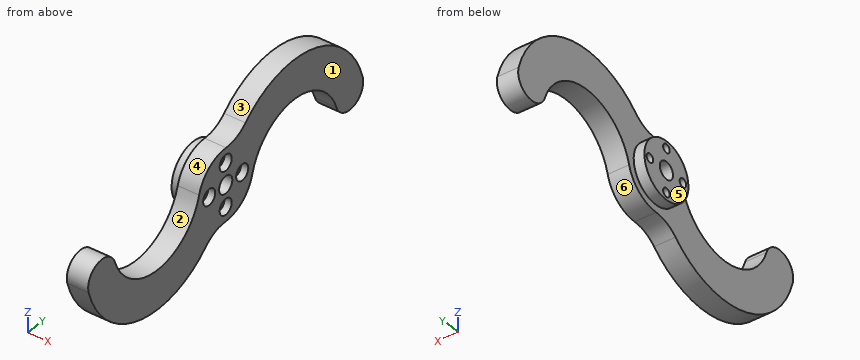
from build123d import *

# Parameters (mm, degrees)
SKETCH1_R                      = 2.4
BOSS_EXTRUDE1_DEPTH            = 6
SKETCH2_R                      = 8
SKETCH2_R_2                    = 2.4
BOSS_EXTRUDE2_DEPTH            = 3
CBORE_FOR_M2_SHCS1_D           = 2.4
CBORE_FOR_M2_SHCS1_CBORE_D     = 4.4
CBORE_FOR_M2_SHCS1_CBORE_DEPTH = 2
FILLET1_R                      = 10


with BuildPart() as part:
    # Sketch1 → Boss-Extrude1 (new body)
    with BuildSketch(Plane(origin=(0, 0, 0), x_dir=(0, 0, -1), z_dir=(1, 0, 0))):
        with BuildLine():
            ThreePointArc((9.139568575, -4.058113633), (9.024618995, 4.307696832), (2.592436286, 9.658119595))
            ThreePointArc((2.592436286, 9.658119595), (-9.251342607, 24.595099021), (1.604842351, 40.264550225))
            ThreePointArc((1.604842351, 40.264550225), (4.773868283, 46.4866715), (-1.367582481, 49.809336247))
            ThreePointArc((-1.367582481, 49.809336247), (-19.682903104, 29.384906165), (-9.139568476, 4.058113857))
            ThreePointArc((-9.139568476, 4.058113857), (-9.024618995, -4.307696832), (-2.592436049, -9.658119658))
            ThreePointArc((-2.592436049, -9.658119658), (9.25134321, -24.595098795), (-1.604841364, -40.264550265))
            ThreePointArc((-1.604841364, -40.264550265), (-4.773867143, -46.486671617), (1.367583702, -49.809336214))
            ThreePointArc((1.367583702, -49.809336214), (19.682903824, -29.384905682), (9.139568575, -4.058113633))
        make_face()
        Circle(SKETCH1_R, mode=Mode.SUBTRACT)
    extrude(amount=BOSS_EXTRUDE1_DEPTH)

    # Sketch2 → Boss-Extrude2 (add)
    with BuildSketch(Plane.ZY):
        Circle(SKETCH2_R)
        Circle(SKETCH2_R_2, mode=Mode.SUBTRACT)
    extrude(amount=BOSS_EXTRUDE2_DEPTH)

    # CBORE for M2 SHCS1 (through all)
    with Locations(Plane(origin=(6, 0, 0), x_dir=(0, 0, -1), z_dir=(1, 0, 0))):
        with Locations((0, -6), (-6, 0), (0, 6), (6, 0)):
            CounterBoreHole(CBORE_FOR_M2_SHCS1_D / 2, CBORE_FOR_M2_SHCS1_CBORE_D / 2, CBORE_FOR_M2_SHCS1_CBORE_DEPTH)

    # Fillet1
    fillet1_edges = [part.edges().sort_by_distance(p)[0] for p in [
        (3, 4.058113857, 9.139568476),
        (3, -4.058113633, -9.139568575),
    ]]
    fillet(fillet1_edges, radius=FILLET1_R)


solid = part.part
The model under review builds one solid part; all positions refer to its coordinate system, in mm. Face numbers are marked on the shaded views. A direction names the side the tool comes from. Round coordinates to 2 decimals unless told otherwise and drop trailing zeros. Order: outer loops, then holes, each group sorted by start corner. A loop starts at its lowest first (then second) coordinate and runs counter-clockwise, first axis right, second up. Notation, with made-up numbers: (87, -14.75) -> (122, -14.75) arc R22 cw to (122, 20.25) -> close; hole circle Ø8 at (82.25, 85). An arc over 180 degrees is marked (long way). Use CSV: the item, a comma, the result in double quotes. Start each with the question number.
(1) Consider section B-B on y = -22. Write out the cut boundary in (x, z).
(2) Insertion check: pin 1 (3 mm diameter, centred on x = 2.5, z = -4.5, fed in from -Y); pin 2 (1.4 mm diameter, centred on y = -6, z = 0, fed in from +X); pin 3 (1.3 mm diameter, centred on y = 0.5, z = -7, fed in from +X); pin 4 (6 mm diameter, centred on y = 12.5, z = 6, fed in from -X). Each pin has a flat end and moves straight along its axis. Give the tip position at first contact, or say it passes through.
(3) Consider section C-C on x = 2.75. State how many separate pieces and enclosed holes the cut face has, and give its area (3 significant figures).
(4) Wall thickness on probe 1 along Y at (x, z) = (3.3, 0); probe 2 along Y at (x, z) = (5.2, -6); probe 3 along Y at (x, z) = (5.25, 0): over which ranges is each line inside the solid? List them lowest first. Write a range as from..to.
(5) Consider section D-D on z = 17. Write out the cut boundary in (x, y).
(6) Mouldability with a two-part tool opening along Y and no side actions: class the marked faces 1, 2 and 3 as pulls with the +Y half, pulls with the -Y half, needs draft (parallel to the pull), parting line crosses it, or undercut.
(7) Consider section A-A on z = -6. Write out the cut boundary in (x, y), and give its area (3 significant figures).
(8) Tool access review of the marked faces 4, 5 and 6: name each direction out of +Z, -Z, +X, -X, +Y, -Y from which nothing blocks a thin tool from reaching the whole face with its end or side.
Responses:
1,outline,"(0, -19.86) -> (6, -19.86) -> (6, -8.95) -> (0, -8.95) -> close"
2,pin 1,"y = -49.29"
2,pin 2,"through"
2,pin 3,"x = 4"
2,pin 4,"x = 0"
3,separate pieces,"1"
3,enclosed holes,"5"
3,area,"1,360 mm²"
4,probe 1,"-50..-39.62, -10.6..-7.2, -4.8..-2.4, 2.4..4.8, 7.2..10.6, 39.62..50"
4,probe 2,"-47.99..-34.79, -15.43..-2.2, 2.2..8"
4,probe 3,"-50..-39.62, -10.6..-8.2, -3.8..-2.4, 2.4..3.8, 8.2..10.6, 39.62..50"
5,outline,"(0, 12.94) -> (6, 12.94) -> (6, 37.22) -> (0, 37.22) -> close"
6,face 1,"needs draft"
6,face 2,"undercut"
6,face 3,"parting line crosses it"
7,outline,"(-3, -5.29) -> (0, -5.29) -> (0, -15.43) -> (6, -15.43) -> (6, -2.2) -> (4, -2.2) -> (4, -1.2) -> (-3, -1.2) -> close; (-3, 1.2) -> (4, 1.2) -> (4, 2.2) -> (6, 2.2) -> (6, 8) -> (0, 8) -> (0, 5.29) -> (-3, 5.29) -> close; (0, -47.99) -> (6, -47.99) -> (6, -34.79) -> (0, -34.79) -> close"
7,area,"226 mm²"
8,face 4,"+Z, +X, -X"
8,face 5,"+Z, -Z, -X, +Y, -Y"
8,face 6,"-Z, +X, -X"
